Check sheet for the modelled part. Datum: model origin and axes. Units: mm. A direction names the side the tool comes from. Round coordinates to 2 decimals unless told otherwise and drop trailing zeros. Loops run counter-clockwise (first coordinate to the right, second up) from the corner with the lowest first, then second, coordinate; pieces in that order, holes last. Notation, with made-up numbers: (20.5, 52.5) - (27.5, 52.5) arc R10 cw to (27.5, 66.5) - close; hole circle Ø10 at (74, 30). An arc over 180 degrees is marked (long way). Put each result on its own line as item: value.
```python
from build123d import *

# Parameters (mm, degrees)
F0_W     = 76.5
F0_H     = 56.5
F1_DEPTH = 25
F2_DEPTH = 3
F0_W_2   = 7
F0_H_2   = 9
F0_R     = 2
F3_DEPTH = 7
F4_DEPTH = 9
F5_DEPTH = 9
F6_DEPTH = 9


with BuildPart() as f1:
    # F0 (on Front) → F1 (new body)
    with BuildSketch(Plane.XZ):
        with Locations((12.333626, 4.463955)):
            Rectangle(F0_W, F0_H)
        Polygon((-22.916374, 20.713955), (-22.916374, 29.713955), (-15.916374, 29.713955), (12.333626, 29.713955), (40.583626, 29.713955), (47.583626, 29.713955), (47.583626, 20.713955), (47.583626, 4.463955), (47.583626, -11.786045), (47.583626, -20.786045), (40.583626, -20.786045), (12.333626, -20.786045), (-15.916374, -20.786045), (-22.916374, -20.786045), (-22.916374, -11.786045), (-22.916374, 4.463955), align=None, mode=Mode.SUBTRACT)
    extrude(amount=F1_DEPTH)

    # F0 (on Front) → F2 (join)
    with BuildSketch(Plane.XZ):
        Polygon((12.333626, 29.713955), (-15.916374, 29.713955), (-15.916374, 20.713955), (-22.916374, 20.713955), (-22.916374, 4.463955), (12.333626, 4.463955), align=None)
        Polygon((40.583626, 29.713955), (12.333626, 29.713955), (12.333626, 4.463955), (47.583626, 4.463955), (47.583626, 20.713955), (40.583626, 20.713955), align=None)
        Polygon((47.583626, 4.463955), (12.333626, 4.463955), (12.333626, -20.786045), (40.583626, -20.786045), (40.583626, -11.786045), (47.583626, -11.786045), align=None)
        Polygon((12.333626, 4.463955), (-22.916374, 4.463955), (-22.916374, -11.786045), (-15.916374, -11.786045), (-15.916374, -20.786045), (12.333626, -20.786045), align=None)
    extrude(amount=F2_DEPTH)

    # F0 (on Front) → F3 (join)
    with BuildSketch(Plane.XZ):
        with Locations((-19.416374, 25.213955)):
            Rectangle(F0_W_2, F0_H_2)
        with Locations((-19.666374, 24.713955)):
            Circle(F0_R, mode=Mode.SUBTRACT)
        with Locations((44.083626, 25.213955)):
            Rectangle(F0_W_2, F0_H_2)
        with Locations((44.333626, 24.713955)):
            Circle(F0_R, mode=Mode.SUBTRACT)
        with Locations((44.083626, -16.286045)):
            Rectangle(F0_W_2, F0_H_2)
        with Locations((44.333626, -15.786045)):
            Circle(F0_R, mode=Mode.SUBTRACT)
        with Locations((-19.416374, -16.286045)):
            Rectangle(F0_W_2, F0_H_2)
        with Locations((-19.666374, -15.786045)):
            Circle(F0_R, mode=Mode.SUBTRACT)
    extrude(amount=F3_DEPTH)

    # F0 (on Front) → F4 (join)
    with BuildSketch(Plane.XZ):
        with Locations((-19.666374, 24.713955)):
            Circle(F0_R)
        with Locations((44.333626, -15.786045)):
            Circle(F0_R)
    extrude(amount=F4_DEPTH)

    # F0 (on Front) → F5 (join)
    with BuildSketch(Plane.XZ):
        with Locations((44.333626, 24.713955)):
            Circle(F0_R)
    extrude(amount=F5_DEPTH)

    # F0 (on Front) → F6 (join)
    with BuildSketch(Plane.XZ):
        with Locations((-19.666374, -15.786045)):
            Circle(F0_R)
    extrude(amount=F6_DEPTH)


solid = f1.part
```
Item 1: Section check D-D on y = -16.5. Enter the section's corners in (x, z).
Filled sheet:
outline: (-25.92, -23.79) - (50.58, -23.79) - (50.58, 32.71) - (-25.92, 32.71) - close; hole (-22.92, -20.79) - (47.58, -20.79) - (47.58, 29.71) - (-22.92, 29.71) - close
Item 2: Tool access check on faces 4 (the flat face through (44, -9, -16)), 5 (the flat face through (12, -12, 32.714)). Record the directions out of +Z, -Z, +X, -X, +Y, -Y that give a thin tool (end or side, any length) a straight path to the whole face; none if there is none.
Filled sheet:
face 4: -Y
face 5: +Z, +X, -X, +Y, -Y
Item 3: Thickness scan on line 1 (Z direction, x = -12, y = -5.25); line 2 (X direction, y = -13.75, z = -4.5); line 3 (Z direction, x = -17.5, y = -6.25). Record the ranges inside material, lowest first. Write a range as from..to.
Filled sheet:
line 1: -23.79..-20.79, 29.71..32.71
line 2: -25.92..-22.92, 47.58..50.58
line 3: -23.79..-11.79, 20.71..32.71
Item 4: Release check for a two-part mould opening along Y. For faces 1 (the flat face through (12, 0, 5)), 2 (the cylindrical face through (42.86, -7.986, 26.066)), 3 (the flat face through (-17.9, -7, 26.3)) record: +Y half, -Y half, draft (parallel to the pull), parting line (faces both ways), or undercut.
Filled sheet:
face 1: +Y half
face 2: draft
face 3: -Y half
Item 5: Section check B-B on z = 28.5. Enter the section's corners in (x, y).
Filled sheet:
outline: (-25.92, -25) - (-22.92, -25) - (-22.92, -7) - (-15.92, -7) - (-15.92, -3) - (40.58, -3) - (40.58, -7) - (47.58, -7) - (47.58, -25) - (50.58, -25) - (50.58, 0) - (-25.92, 0) - close
Item 6: Section check C-C on x = 14. Enter the section's corners in (y, z), then the cut area to 4 significant figures.
Filled sheet:
outline: (-25, -23.79) - (0, -23.79) - (0, 32.71) - (-25, 32.71) - (-25, 29.71) - (-3, 29.71) - (-3, -20.79) - (-25, -20.79) - close
area: 301.5 mm²
Item 7: Section check A-A on y = -4.25. Enter the section's corners in (x, z), then the cut area to 3 significant figures.
Filled sheet:
outline: (-25.92, -23.79) - (50.58, -23.79) - (50.58, 32.71) - (-25.92, 32.71) - close; hole (-22.92, -11.79) - (-15.92, -11.79) - (-15.92, -20.79) - (40.58, -20.79) - (40.58, -11.79) - (47.58, -11.79) - (47.58, 20.71) - (40.58, 20.71) - (40.58, 29.71) - (-15.92, 29.71) - (-15.92, 20.71) - (-22.92, 20.71) - close
area: 1,010 mm²
Item 8: Go/stop test with a flat-tipped pin: pin 1 (7.5 mm diameter, centred on x = 43.5, z = 25.5, fed in from -Y). Record where the tip stops, or that it passes through.
Filled sheet:
pin 1: y = -9
